Can you work these out from the model? Positions are in its coordinate system, mm. A direction names the side the tool comes from. Give positions to 0.01 mm unless a question says otherwise; leave off trailing zeros. Write each loop counter-clockwise with the first axis right and the second up, starting at its lowest first coordinate (ties: lowest second). Pieces come first, ordered by that corner, then holes. Notation, with made-up numbers: (14, -36.75) -> (70, -36.75) arc R11 ccw to (70, -17.75) -> close; hole circle Ø10 at (38.5, 52). An arc over 180 degrees is marked (long way). Answer as CSV lines item,"result". Start each with the question number.
1. On a 3-axis mill with a long thin cutter (end or side, diameter ignored), from which of +Z, -Z, +X, -X, +Y, -Y can I reach the whole of each face in a straight line? I mean faces 4 (the face through (15.349, 1.565, -28.504)), 5 (the face through (14, 2, -63.5)). Say none if no direction works.
2. If we section it at B-B on z = 0: Write out the boundary of the cut face in (x, y) (3 decimals), plus the area to 3 significant figures.
3. If we section it at D-D on z = -50.8: Write out the boundary of the cut face in (x, y) (1 decimal).
4. I need wall thicknesses on line 1 (X direction, y = 1.2, z = -25.4); line 2 (Z direction, x = 50.8, y = 1.05); line 3 (X direction, y = 0.3, z = -15). Which ranges of each line are inside material? Lowest first, please. Write a range as [from, to].
5. I'm going to push flat-ended pins straight in: P1, Ø6.5, axis at x = 25.4, z = 25.4, coming from the +Y side (3 decimals); P2, Ø1.5, axis at y = 3, z = -35.5, coming from the -X side; P3, Ø1.6, axis at y = 1, z = 1.5, coming from the -X side. Where does each tip first touch, or does it pass through?
6. If we mould it in two halves opening along Z, with no side actions, what happens to faces 1 (the face through (23.152, 1.565, 29.598)), 2 (the face through (14, 3.175, -15)), 3 (the face through (19.216, 1.565, -26.132))? For each: pulls with the +Z half, pulls with the -Z half, needs draft (parallel to the pull), parting line crosses it, or undercut.
7. If we section it at A-A on x = 0: Write out the boundary of the cut face in (y, z) (3 decimals), plus the area to 3 significant figures.
8. If we section it at C-C on x = 12.5: Write out the boundary of the cut face in (y, z) (3 decimals), plus the area to 3 significant figures.
```python
from build123d import *

# Parameters (mm, degrees)
SKETCH1_W                  = 127
SKETCH1_H                  = 127
BOSS_EXTRUDE_1_DEPTH       = 3.175
SKETCH5_R                  = 2.5273
SKETCH5_R_2                = 2.0193
CUT_EXTRUDE1_DEPTH         = 90.858670283
FILLET1_R                  = 6.35
FILLET2_R                  = 6.35
FILLET3_R                  = 6.35
F_10_CLEARANCE_HOLE1_D     = 5.1054
F_10_CLEARANCE_HOLE1_DEPTH = 9.906
F_10_CLEARANCE_HOLE1_TIP   = 1.533816902


with BuildPart() as part:
    # Sketch1 → Boss-Extrude 1 (new body)
    with BuildSketch(Plane(origin=(0, 0, 0), x_dir=(1, 0, 0), z_dir=(0, 1, 0))):
        Rectangle(SKETCH1_W, SKETCH1_H)
    extrude(amount=BOSS_EXTRUDE_1_DEPTH)

    # Sketch5 → Cut-Extrude1 (cut, through all)
    with BuildSketch(Plane.XZ):
        with BuildLine():
            ThreePointArc((-30.1625, -25.4), (-29.613538389, -23.180202601), (-28.093208455, -21.472146328))
            ThreePointArc((-28.093208455, -21.472146328), (-27.35728191, -20.769991802), (-26.881161446, -19.871149123))
            Line((-26.881161446, -19.871149123), (-17.158114653, 8.86613294))
            ThreePointArc((-17.158114653, 8.86613294), (-12.122211864, 12.122211864), (-8.86613294, 17.158114653))
            Line((-8.86613294, 17.158114653), (19.871149123, 26.881161446))
            ThreePointArc((19.871149123, 26.881161446), (20.769991802, 27.35728191), (21.472146328, 28.093208455))
            ThreePointArc((21.472146328, 28.093208455), (23.180202601, 29.613538389), (25.4, 30.1625))
            Line((25.4, 30.1625), (63.5, 34.925))
            Line((63.5, 34.925), (63.5, 63.5))
            Line((63.5, 63.5), (-63.5, 63.5))
            Line((-63.5, 63.5), (-63.5, -63.5))
            Line((-63.5, -63.5), (-34.925, -63.5))
            Line((-34.925, -63.5), (-30.1625, -25.4))
        make_face()
        with BuildLine():
            ThreePointArc((16.821574871, -28.281660245), (19.229977614, -26.085792739), (18.434943467, -22.925071528))
            Line((18.434943467, -22.925071528), (-7.573712289, 3.083584229))
            ThreePointArc((-7.573712289, 3.083584229), (-10.541284963, 3.930219773), (-12.826295631, 1.856092108))
            Line((-12.826295631, 1.856092108), (-20.866122824, -21.906292943))
            ThreePointArc((-20.866122824, -21.906292943), (-21.033571343, -22.90957249), (-20.875162107, -23.914318912))
            ThreePointArc((-20.875162107, -23.914318912), (-20.697290849, -24.647714886), (-20.6375, -25.4))
            ThreePointArc((-20.6375, -25.4), (-19.70756403, -27.64506403), (-17.4625, -28.575))
            Line((-17.4625, -28.575), (13.902307909, -28.575))
            ThreePointArc((13.902307909, -28.575), (15.369291874, -28.501480873), (16.821574871, -28.281660245))
        make_face()
        with BuildLine():
            ThreePointArc((28.281660245, -16.821574871), (28.501480873, -15.369291874), (28.575, -13.902307909))
            Line((28.575, -13.902307909), (28.575, 17.4625))
            ThreePointArc((28.575, 17.4625), (27.64506403, 19.70756403), (25.4, 20.6375))
            ThreePointArc((25.4, 20.6375), (24.647714886, 20.697290849), (23.914318912, 20.875162107))
            ThreePointArc((23.914318912, 20.875162107), (22.90957249, 21.033571343), (21.906292943, 20.866122824))
            Line((21.906292943, 20.866122824), (-1.856092108, 12.826295631))
            ThreePointArc((-1.856092108, 12.826295631), (-3.930219773, 10.541284963), (-3.083584229, 7.573712289))
            Line((-3.083584229, 7.573712289), (22.925071528, -18.434943467))
            ThreePointArc((22.925071528, -18.434943467), (26.085792739, -19.229977614), (28.281660245, -16.821574871))
        make_face()
        with Locations(Location((25.4, -25.4, 0), (0, 0, 270))):
            Circle(SKETCH5_R)
        with Locations(Location((-25.4, -25.4, 0), (0, 0, 270))):
            Circle(SKETCH5_R_2)
        with Locations(Location((25.4, 25.4, 0), (0, 0, 270))):
            Circle(SKETCH5_R_2)
    extrude(amount=-CUT_EXTRUDE1_DEPTH, mode=Mode.SUBTRACT)

    # Fillet1
    fillet1_edges = [part.edges().sort_by_distance(p)[0] for p in [
        (63.5, 1.5875, -63.5),
    ]]
    fillet(fillet1_edges, radius=FILLET1_R)

    # Fillet2
    fillet2_edges = [part.edges().sort_by_distance(p)[0] for p in [
        (-34.925, 1.5875, -63.5),
        (63.5, 1.5875, 34.925),
    ]]
    fillet(fillet2_edges, radius=FILLET2_R)

    # Fillet3
    fillet3_edges = [part.edges().sort_by_distance(p)[0] for p in [
        (-8.86613294, 1.5875, 17.158114653),
        (-17.158114653, 1.5875, 8.86613294),
    ]]
    fillet(fillet3_edges, radius=FILLET3_R)

    # #10 Clearance Hole1
    with Locations(Plane(origin=(0, 0, 0), x_dir=(-1, 0, 0), z_dir=(0, -1, 0))):
        with Locations((-50.8, 50.8), (-25.4, 50.8), (38.1, 50.8), (50.8, 50.8), (0, 50.8), (76.2, 50.8), (25.4, 50.8), (-50.8, 25.4), (-50.8, 0), (-50.8, -25.4), (-50.8, -50.8), (-50.8, -76.2)):
            Hole(F_10_CLEARANCE_HOLE1_D / 2, depth=F_10_CLEARANCE_HOLE1_DEPTH)
            with Locations((0, 0, -(F_10_CLEARANCE_HOLE1_DEPTH + F_10_CLEARANCE_HOLE1_TIP / 2))):  # 118° drill point
                Cone(0, F_10_CLEARANCE_HOLE1_D / 2, F_10_CLEARANCE_HOLE1_TIP, mode=Mode.SUBTRACT)


solid = part.part
```
Computed values:
1,face 4,"+Y, -Y"
1,face 5,"-Z, +X, -X, +Y, -Y"
2,outline,"(-20.158, 0) -> (-13.454, 0) -> (-13.454, 3.175) -> (-20.158, 3.175) -> close; (-4.49, 0) -> (4.49, 0) -> (4.49, 3.175) -> (-4.49, 3.175) -> close; (28.575, 0) -> (48.247, 0) -> (48.247, 3.175) -> (28.575, 3.175) -> close; (53.353, 0) -> (63.5, 0) -> (63.5, 3.175) -> (53.353, 3.175) -> close"
2,area,"144 mm2"
3,outline,"(-33.3, 0) -> (-28, 0) -> (-28, 3.2) -> (-33.3, 3.2) -> close; (-22.8, 0) -> (-2.6, 0) -> (-2.6, 3.2) -> (-22.8, 3.2) -> close; (2.6, 0) -> (22.8, 0) -> (22.8, 3.2) -> (2.6, 3.2) -> close; (28, 0) -> (48.2, 0) -> (48.2, 3.2) -> (28, 3.2) -> close; (53.4, 0) -> (63.5, 0) -> (63.5, 3.2) -> (53.4, 3.2) -> close"
4,line 1,"x = [-30.16, -27.42], [-23.38, -20.64], [19.36, 22.87], [27.93, 48.25], [53.35, 63.5]"
4,line 2,"z = [-63.5, -53.35], [-48.25, -27.95], [-22.85, -2.55], [2.55, 22.85], [27.95, 33.34]"
4,line 3,"x = [-25.23, -18.53], [10.51, 19.49], [28.53, 63.5]"
5,P1,"stops at y = 3.175"
5,P2,"stops at x = -31.52"
5,P3,"stops at x = -19.92"
6,face 1,"pulls with the +Z half"
6,face 2,"needs draft"
6,face 3,"undercut"
7,outline,"(0, -63.5) -> (3.175, -63.5) -> (3.175, -53.353) -> (0, -53.353) -> close; (0, -48.247) -> (3.175, -48.247) -> (3.175, -28.575) -> (0, -28.575) -> close; (0, -4.49) -> (3.175, -4.49) -> (3.175, 4.49) -> (0, 4.49) -> close; (0, 13.454) -> (3.175, 13.454) -> (3.175, 20.158) -> (0, 20.158) -> close"
7,area,"144 mm2"
8,outline,"(0, -63.5) -> (3.175, -63.5) -> (3.175, -28.575) -> (0, -28.575) -> close; (0, -16.99) -> (3.175, -16.99) -> (3.175, -8.01) -> (0, -8.01) -> close; (0, 17.684) -> (3.175, 17.684) -> (3.175, 24.387) -> (0, 24.387) -> close"
8,area,"161 mm2"
